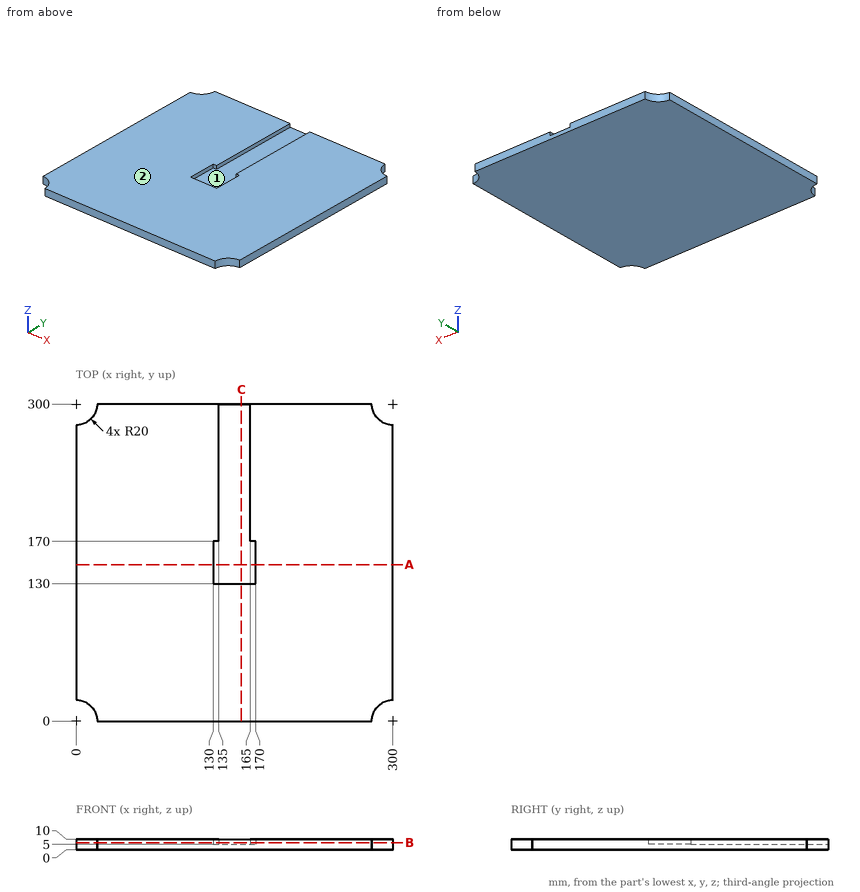
Here's the drawing with two shaded views (mm, measured from the low corner). I have some questions. Coordinates: 2 decimals unless noted, no trailing zeros. Write each loop counter-clockwise with the first axis right and the second up, starting at its lowest first coordinate (ties: lowest second). Pieces come first, ordered by that corner, then holes.
Item 1: I want a section at A-A on y = 148. Write out the boundary of the cut face in (x, z), and give its area (3 significant figures).
Item 2: I want a section at B-B on z = 6.5. Write out the boundary of the cut face in (x, y), and give its area (3 significant figures).
Item 3: If I drill on line 1 (X direction, y = 274.5, z = 8.5); line 2 (X direction, y = 156, z = 7); line 3 (Y direction, x = 151, z = 9.25), over which ranges is the centre line in solid material (lowest first)?
Item 4: I want a section at C-C on x = 156.5. Write out the boundary of the cut face in (y, z), and give its area (3 significant figures).
Item 5: If we mould it in two halves opening along X, with no side actions, what happens to the marked faces 1 and 2? For each: +X half, -X half, draft (parallel to the pull), parting line (faces both ways), or undercut.
Item 6: Will this pin go through, and if not, where does the flat tip stop? pin 1 (2.5 mm diameter, centred on x = 146.5, z = 8, fed in from +Y).
Findings below:
1. outline: (0, 0) - (300, 0) - (300, 10) - (170, 10) - (170, 5) - (130, 5) - (130, 10) - (0, 10) - close
1. area: 2,800 mm2
2. outline: (0, 20) arc R20 cw to (20, 0) - (280, 0) arc R20 cw to (300, 20) - (300, 280) arc R20 cw to (280, 300) - (165, 300) - (165, 170) - (170, 170) - (170, 130) - (130, 130) - (130, 170) - (135, 170) - (135, 300) - (20, 300) arc R20 cw to (0, 280) - close
2. area: 83,200 mm2
3. line 1: x = 0 to 135, 165 to 300
3. line 2: x = 0 to 130, 170 to 300
3. line 3: y = 0 to 130
4. outline: (0, 0) - (300, 0) - (300, 5) - (130, 5) - (130, 10) - (0, 10) - close
4. area: 2,150 mm2
5. face 1: undercut
5. face 2: draft
6. pin 1: stops at y = 130
